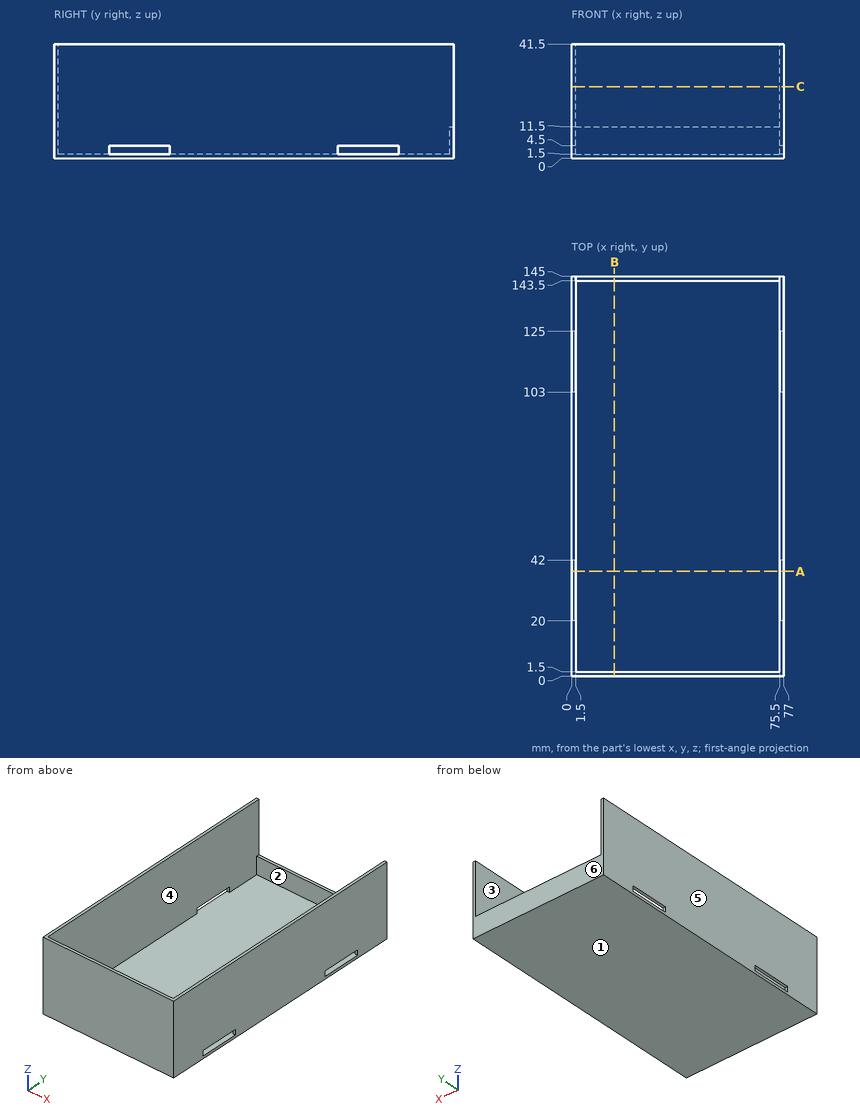
Input: dimensioned drawing with shaded views. Units: mm. Origin: part minimum x, y, z. A direction names the side the tool comes from. Give positions to 0.01 mm unless a question says otherwise; leave off trailing zeros. Write each loop counter-clockwise with the first axis right and the second up, starting at its lowest first coordinate (ties: lowest second). Pieces come first, ordered by that corner, then holes. Notation, with made-up numbers: (89, 5) - (105, 5) arc R14 ccw to (105, 31) - close; hole circle Ø11 at (63, 2.5). An arc over 180 degrees is marked (long way). One line per item, written item: value. Start each with the question number.
Q1. Set-up query: the marked faces 1 and 2. Return all of +Z, -Z, +X, -X, +Y, -Y with unobstructed straight access to the full face (end or side cutting, diameter ignored); none if empty.
Q2. Draft query along X for the marked faces 3, 4, 5 and 6. Return one class per face: +X half, -X half, draft (parallel to the pull), parting line (faces both ways), or undercut.
Q3. First-contact query: pin 1 Ø2 at (y, z) = (125, 36.5) entering from -X; pin 2 Ø1.5 at (x, z) = (26.5, 20) entering from +Y; pin 3 Ø3 at (x, y) = (24.5, 129) entering from +Z; pin 4 Ø1.6 at (x, y) = (33.5, 144) entering from +Z. Flat tips, straight axial feed; report the tip coordinate or a pass-through.
Q4. Section query A-A, the plane y = 38. Return the cut outline in (x, z).
Q5. Section query B-B, the plane x = 15.5. Return the cut outline in (y, z).
Q6. Section query C-C, the plane z = 26. Return the cut outline in (x, y).
Q7. Material intervals for probe 1 along Y at (x, z) = (54, 10.5); probe 2 along X at (y, z) = (127.5, 22); probe 3 along Z at (x, y) = (62, 69.5), sorted ascending. Write a range as from..to.
Answer:
1. face 1: -Z, +X, -X, +Y, -Y
1. face 2: +Z
2. face 3: undercut
2. face 4: undercut
2. face 5: -X half
2. face 6: draft
3. pin 1: stops at x = 0
3. pin 2: stops at y = 1.5
3. pin 3: stops at z = 1.5
3. pin 4: stops at z = 11.5
4. outline: (0, 0) - (77, 0) - (77, 1.5) - (0, 1.5) - close; (0, 4.5) - (1.5, 4.5) - (1.5, 41.5) - (0, 41.5) - close; (75.5, 4.5) - (77, 4.5) - (77, 41.5) - (75.5, 41.5) - close
5. outline: (0, 0) - (145, 0) - (145, 11.5) - (143.5, 11.5) - (143.5, 1.5) - (1.5, 1.5) - (1.5, 41.5) - (0, 41.5) - close
6. outline: (0, 0) - (77, 0) - (77, 145) - (75.5, 145) - (75.5, 1.5) - (1.5, 1.5) - (1.5, 145) - (0, 145) - close
7. probe 1: y = 0..1.5, 143.5..145
7. probe 2: x = 0..1.5, 75.5..77
7. probe 3: z = 0..1.5
